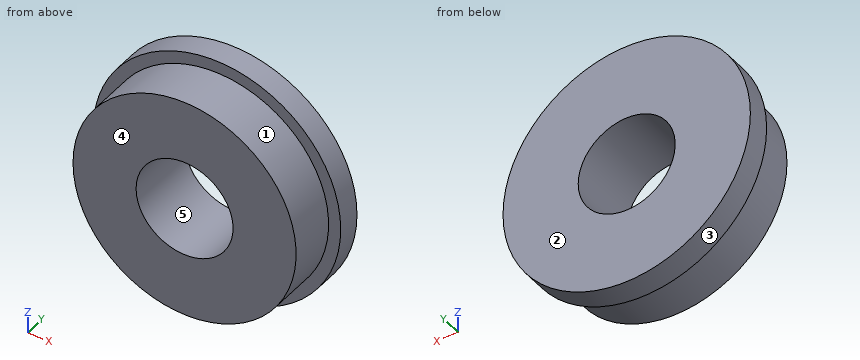
Autodesk Inventor part; units mm, degrees
ref_plane "YZ Plane" through (0, 0, 0) normal (1, 0, 0) x (0, 1, 0)
ref_plane "XZ Plane" through (0, 0, 0) normal (0, 1, 0) x (-1, 0, 0)
ref_plane "XY Plane" through (0, 0, 0) normal (0, 0, 1) x (1, 0, 0)
sketch "Эскиз1" plane through (0, 0, 0) normal (0, 1, 0) x (-1, 0, 0)
  circle A0 centre (0, -0.3241) radius 4.6
  circle A1 centre (0, -0.3241) radius 2
  point P0 (0, 0)
  dimension "d0" = 9.2
  dimension "d1" = 4
extrude "Выдавливание1" add sketch "Эскиз1" along normal blind 2
sketch "Эскиз2" plane through (0, 2, -0.3241) normal (0, 1, 0) x (1, 0, 0)
  circle A0 centre (0, 0) radius 5.1
  point P0 (0, -0.3241)
  dimension "d4" = 10.2
extrude "Выдавливание2" add sketch "Эскиз2" along normal blind 1
sketch "Эскиз3" plane through (0, 2, -0.3241) normal (0, -1, 0) x (1, 0, 0)
  circle A0 centre (0, 0) radius 2
  point P0 (0, 0.3241)
  dimension "d7" = 4
extrude "Выдавливание3" cut sketch "Эскиз3" against normal blind 1
properties part number "bearing"
Check sheet for the modelled part. Datum: model origin and axes. Units: mm. Face numbers are marked on the shaded views. A direction names the side the tool comes from. Round coordinates to 2 decimals unless told otherwise and drop trailing zeros. Write each loop counter-clockwise with the first axis right and the second up, starting at its lowest first coordinate (ties: lowest second). Pieces come first, ordered by that corner, then holes. Notation, with made-up numbers: (34.25, -33) -> (66.25, -33) arc R13 ccw to (66.25, -8) -> close; hole circle Ø7 at (-8.5, -33.75). An arc over 180 degrees is marked (long way). One line per question, with ' | ' between items. Start each with the question number.
1. Sectioned sample at B-B, the plane z = 0.75. Record the cut outline in (x, y).
2. Depth check by flat-ended pin: pin 1 (1.5 mm diameter, centred on x = 3, y = 2, fed in from -Z). Enter the tip coordinate at first touch or a pass-through.
3. Release check for a two-part mould opening along Z. For the marked faces 3, 4 and 5 record: +Z half, -Z half, draft (parallel to the pull), parting line (faces both ways), or undercut.
4. Scan lines: line 1 along Z through (x, y) = (0, 1.7); line 2 along Z through (x, y) = (0, 2.2); line 3 along Y through (x, z) = (2, -4.5). Record each from-to range of solid material in increasing order. Write a range as from..to.
5. Sectioned sample at A-A, the plane x = 0. Record the cut outline in (y, z), then the cut area to 3 significant figures.
6. Sectioned sample at D-D, the plane y = 0.65. Record the cut outline in (x, z).
7. Sectioned sample at C-C, the plane z = -4.5. Record the cut outline in (x, y).
8. Set-up check for the marked faces 1 and 2: record each of +Z, -Z, +X, -X, +Y, -Y from which the full face is reachable in a straight line by a thin tool's end or side.
Taken from the geometry:
1) outline: (-4.99, 2) -> (-4.47, 2) -> (-4.47, 0) -> (-1.69, 0) -> (-1.69, 3) -> (-4.99, 3) -> close; (1.69, 0) -> (4.47, 0) -> (4.47, 2) -> (4.99, 2) -> (4.99, 3) -> (1.69, 3) -> close
2) pin 1: stops at z = -4.9
3) face 3: parting line | face 4: draft | face 5: undercut
4) line 1: z = -4.92..-2.32, 1.68..4.28 | line 2: z = -5.42..-2.32, 1.68..4.78 | line 3: y = 2..3
5) outline: (0, -4.92) -> (2, -4.92) -> (2, -5.42) -> (3, -5.42) -> (3, -2.32) -> (0, -2.32) -> close; (0, 1.68) -> (3, 1.68) -> (3, 4.78) -> (2, 4.78) -> (2, 4.28) -> (0, 4.28) -> close | area: 16.6 mm^2
6) outline: circle Ø9.2 at (0, -0.32); hole circle Ø4 at (0, -0.32)
7) outline: (-2.93, 2) -> (-1.93, 2) -> (-1.93, 0) -> (1.93, 0) -> (1.93, 2) -> (2.93, 2) -> (2.93, 3) -> (-2.93, 3) -> close
8) face 1: -Y | face 2: +Z, -Z, +X, -X, +Y
